Geometry check sheet. Reference: the model listing, model coordinates, mm. Face numbers are marked on the shaded views. A direction names the side the tool comes from. Coordinates: 2 decimals unless noted, no trailing zeros. Write each loop counter-clockwise with the first axis right and the second up, starting at its lowest first coordinate (ties: lowest second). Pieces come first, ordered by that corner, then holes. Notation, with made-up numbers: M -33,39 L -28,39 A21 ccw -28,71 Z; hole C -31.75,-20 d7. An arc over 180 degrees is marked long. Write item = value, one per line. Start each with the question number.
```python
from build123d import *

# Parameters (mm, degrees)
SKETCH1_W           = 35
SKETCH1_H           = 15
BOSS_EXTRUDE1_DEPTH = 12
SHELL1_T            = -2.5
FILLET1_R           = 0.5
SKETCH3_W           = 30
SKETCH3_H           = 10
CUT_EXTRUDE1_DEPTH  = 0.5


with BuildPart() as part:
    # Sketch1 → Boss-Extrude1 (new body)
    with BuildSketch(Plane(origin=(0, 0, 0), x_dir=(1, 0, 0), z_dir=(0, 1, 0))):
        with Locations((17.5, 7.5)):
            Rectangle(SKETCH1_W, SKETCH1_H)
    extrude(amount=BOSS_EXTRUDE1_DEPTH)

    # Shell1
    shell1_openings = [part.faces().sort_by_distance(p)[0] for p in [
        (17.5, 12, -7.5),
    ]]
    offset(amount=SHELL1_T, openings=shell1_openings, kind=Kind.INTERSECTION)

    # Fillet1
    fillet1_edges = [part.edges().sort_by_distance(p)[0] for p in [
        (35, 12, -7.5),
        (17.5, 12, -15),
        (0, 12, -7.5),
        (17.5, 0, -15),
        (35, 0, -7.5),
        (17.5, 0, 0),
        (0, 0, -7.5),
        (17.5, 12, 0),
        (0, 6, -15),
        (35, 6, -15),
        (35, 6, 0),
        (0, 6, 0),
    ]]
    fillet(fillet1_edges, radius=FILLET1_R)

    # Sketch3 → Cut-Extrude1 (cut)
    with BuildSketch(Plane(origin=(0, 2.5, 0), x_dir=(1, 0, 0), z_dir=(0, 1, 0))):
        with Locations((17.5, 7.5)):
            Rectangle(SKETCH3_W, SKETCH3_H)
    extrude(amount=-CUT_EXTRUDE1_DEPTH, mode=Mode.SUBTRACT)


solid = part.part
```
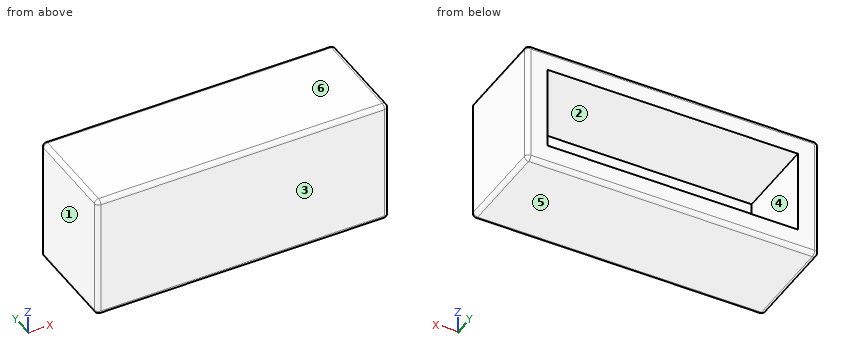
Q1. Scan lines: L1, parallel to Z at x = 5, y = 3.75; L2, parallel to X at y = 5, z = -10.75; L3, parallel to Y at x = 20.5, z = -11.25. Record each from-to range of solid material in increasing order.
Q2. Set-up check for the marked faces 1 and 2: record each of +Z, -Z, +X, -X, +Y, -Y from which the full face is reachable in a straight line by a thin tool's end or side.
Q3. Gauge pin test, flat end, axial feed: pin 1 (5 mm diameter, centred on x = 22.5, z = -4.5, fed in from +Y). Record the tip position at first contact, or that the pin passes through.
Q4. Draft check along Z on the marked faces 3, 4, 5 and 6. Enter one of: pulls with the +Z half, pulls with the -Z half, needs draft (parallel to the pull), parting line crosses it, or undercut.
Q5. Cross-section at A-A on y = 3. Enter the section's corners in (x, z).
Q6. Cross-section at B-B on x = 19. Enter the section's corners in (y, z), and give its area (3 significant figures).
Q7. Cross-section at C-C on z = -10.5. Enter the section's corners in (x, y), and give its area (3 significant figures).
Values found:
q1.L1 = -15 to -12.5, -2.5 to 0
q1.L2 = 0 to 2.5, 32.5 to 35
q1.L3 = 0 to 2
q2.face_1 = +Z, -Z, -X, +Y, -Y
q2.face_2 = +Y
q3.pin_1 = 12
q4.face_3 = needs draft
q4.face_4 = undercut
q4.face_5 = pulls with the -Z half
q4.face_6 = pulls with the +Z half
q5.outline = M 0,-14.5 A0.5 ccw 0.5,-15 L 34.5,-15 A0.5 ccw 35,-14.5 L 35,-0.5 A0.5 ccw 34.5,0 L 0.5,0 A0.5 ccw 0,-0.5 Z; hole M 2.5,-12.5 L 32.5,-12.5 L 32.5,-2.5 L 2.5,-2.5 Z
q6.outline = M 0,-14.5 A0.5 ccw 0.5,-15 L 11.5,-15 A0.5 ccw 12,-14.5 L 12,-12.5 L 2,-12.5 L 2,-2.5 L 12,-2.5 L 12,-0.5 A0.5 ccw 11.5,0 L 0.5,0 A0.5 ccw 0,-0.5 Z
q6.area = 79.8 mm²
q7.outline = M 0,0.5 A0.5 ccw 0.5,0 L 34.5,0 A0.5 ccw 35,0.5 L 35,11.5 A0.5 ccw 34.5,12 L 32.5,12 L 32.5,2 L 2.5,2 L 2.5,12 L 0.5,12 A0.5 ccw 0,11.5 Z
q7.area = 120 mm²
